Print and shaded views of the part. All mm, measured from the part's lowest x, y and z. A direction names the side the tool comes from. Coordinates: 2 decimals unless noted, no trailing zeros. Order: outer loops, then holes, each group sorted by start corner. A loop starts at its lowest first (then second) coordinate and runs counter-clockwise, first axis right, second up. Notation, with made-up numbers: (10.5, 9.25) -> (40.5, 9.25) arc R9 cw to (40.5, 21.25) -> close; hole circle Ø11 at (36.25, 70). An arc over 180 degrees is marked (long way). Return JSON: item names as keys, results as strings. Group by question number.
1) Cut at A-A (y = 3). Write the cut outline in (x, z), and give its area (3 significant figures).
2) Cut at C-C (x = 5). Write the cut outline in (y, z).
3) Cut at B-B (x = 13). Write the cut outline in (y, z).
4) Which spindle directions (+Z, -Z, +X, -X, +Y, -Y) get a long thin tool onto all of the face, cutting with end or side? Do the marked faces 1 and 2. Say none if no direction does.
5) Cut at D-D (z = 5.25). Write the cut outline in (x, y), and give its area (3 significant figures).
6) Probe line 1 (Y direction, x = 18, z = 4.5); line 2 (X direction, y = 3.4, z = 4.5); line 3 (Z direction, x = 13, y = 2.95). List the from-to ranges inside material, lowest first.
7) Flat gauge pins, fed straight in: pin 1 (1 mm diameter, centred on x = 13.5, z = 1, fed in from -Y); pin 2 (1 mm diameter, centred on x = 10, y = 0.5, fed in from -Z); pin 3 (1.3 mm diameter, centred on y = 3.5, z = 4, fed in from -X); pin 4 (1 mm diameter, centred on y = 1.5, z = 0.5, fed in from -X). Where does each tip first touch, or does it go through?
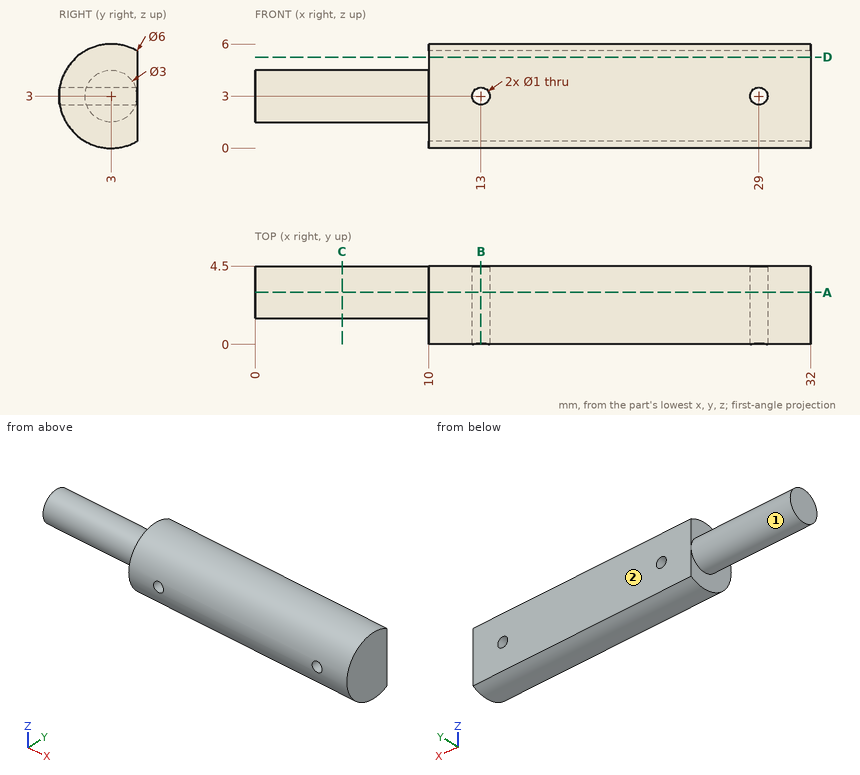
Answers below:
{
 "1": {"outline": "(0, 1.5) -> (10, 1.5) -> (10, 0) -> (32, 0) -> (32, 6) -> (10, 6) -> (10, 4.5) -> (0, 4.5) -> close; hole circle Ø1 at (13, 3); hole circle Ø1 at (29, 3)", "area": "160 mm^2"},
 "2": {"outline": "circle Ø3 at (3, 3)"},
 "3": {"outline": "(0.04, 2.5) arc R3 ccw to (4.5, 0.4) -> (4.5, 2.5) -> close; (0.04, 3.5) -> (4.5, 3.5) -> (4.5, 5.6) arc R3 ccw to start"},
 "4": {"face 1": "-X", "face 2": "+Z, -Z, +X, -X, +Y"},
 "5": {"outline": "(10, 1.02) -> (32, 1.02) -> (32, 4.5) -> (10, 4.5) -> close", "area": "76.7 mm^2"},
 "6": {"line 1": "y = 0.4 to 4.5", "line 2": "x = 10 to 32", "line 3": "z = 0 to 2.5, 3.5 to 6"},
 "7": {"pin 1": "stops at y = 0.4", "pin 2": "stops at z = 0.76", "pin 3": "stops at x = 0", "pin 4": "stops at x = 10"}
}
